Autodesk Fusion 360 part; units mm, degrees
sketch "Sketch1" plane through (0, 0, 0) normal (0, 0, 1) x (1, 0, 0)
  line L0 (0, 0) -> (0, 60.4496)
  line L1 (0, 60.4496) -> (70, 60.4496)
  line L2 (70, 60.4496) -> (90, 40)
  line L3 (90, 40) -> (130, 40)
  line L4 (130, 40) -> (138.9297, 30.8696)
  line L5 (138.9297, 30.8696) -> (163.3358, 30.8696)
  line L6 (200, 0) -> (0, 0)
  line L7 (260, 0) -> (200, 0)
  line L8 (180, 20) -> (190, 20)
  line L9 (190, 20) -> (190, 30.8696)
  line L10 (190, 30.8696) -> (206.2856, 30.8696)
  line L11 (206.2856, 30.8696) -> (240, 20)
  line L12 (240, 20) -> (284.6944, 20)
  line L13 (284.6944, 20) -> (290, 20)
  line L14 (260, 0) -> (290, 0)
  line L15 (290, 0) -> (290, 20)
  line L16 (180, 20) -> (180, 30.8696)
  line L17 (180, 30.8696) -> (163.3358, 30.8696)
revolve "Revolve1" add sketch "Sketch1" angle 360 about axis through (260, 0, 0) along (-1, 0, 0)
hole "Hole1" at (290, 0, 0) direction (-1, 0, 0) diameter 20 depth 20 tip angle 118
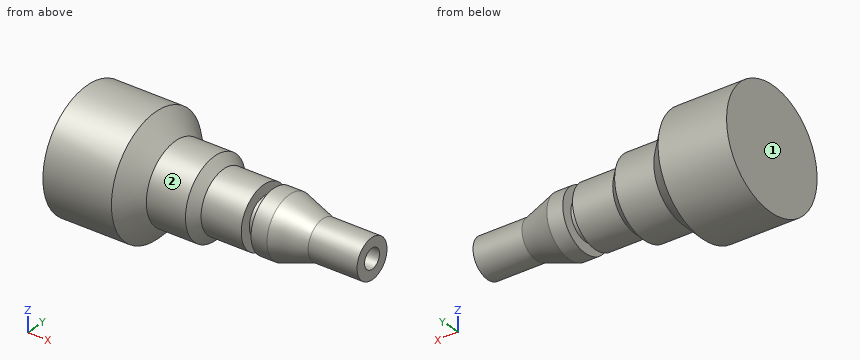
CAD build for the part. Positions are in the model's coordinates, mm. Face numbers are marked on the shaded views. A direction names the side the tool comes from. Give positions to 0.01 mm unless a question says otherwise; leave off trailing zeros. Order: outer loops, then holes, each group sorted by start corner. A loop starts at its lowest first (then second) coordinate and runs counter-clockwise, first axis right, second up. Notation, with made-up numbers: (87, -14.75) - (103, -14.75) arc R23 ccw to (103, 8.25) - close; hole circle Ø10 at (-13, -38.5). An arc over 180 degrees is marked (long way). Write each question's results on one line, items separated by ' | '.
1. Pin check, flat tips, straight feed: pin 1 (3 mm diameter, centred on x = 234, z = 7, fed in from +Y); pin 2 (5 mm diameter, centred on x = 235, z = -21, fed in from +Y); pin 3 (12 mm diameter, centred on y = 38, z = -4, fed in from +X). Stop position of each tip, or through.
Calculated:
pin 1: stops at y = 21.47 | pin 2: stops at y = 11.46 | pin 3: stops at x = 137.62
2. Saw through at A-A on x = 40.5. List the corners of the cut face in (y, z), and give its area (3 significant figures).
Calculated:
outline: circle Ø120.9 at (0, 0) | area: 11,500 mm2
3. 3-axis set-ups, long thin cutter, end or side, ignore diameter. For the marked faces 1 and 2: which of +Z, -Z, +X, -X, +Y, -Y reach the whole face in a straight line?
Calculated:
face 1: +Z, -Z, -X, +Y, -Y | face 2: +X
4. Probe L1, parallel to Y at x = 279, z = 0; L2, parallel to Y at x = 111, z = 1.5. List the from-to ranges inside material, lowest first. Write a range as from..to.
Calculated:
L1: y = -20..-10, 10..20 | L2: y = -39.97..39.97
